Read the model definition and answer for the solid it produces. Units are mm, in the model's axes. A direction names the side the tool comes from. Coordinates: 2 decimals unless noted, no trailing zeros. Loops run counter-clockwise (first coordinate to the right, second up) from the corner with the lowest first, then second, coordinate; pieces in that order, holes last. Notation, with made-up numbers: (62.5, 75) -> (110.5, 75) arc R28 ccw to (110.5, 108) -> close; hole circle Ø6 at (4, 2). An arc over 180 degrees is marked (long way). Answer in a Markdown table with one row per item.
```python
from build123d import *

# Parameters (mm, degrees)
EXTRUDE_1_DEPTH = 6.5
SKETCH_2_R      = 8.75
EXTRUDE_2_DEPTH = 3
SKETCH_3_R      = 10
EXTRUDE_3_DEPTH = 12.5
CHAMFER_1_SIZE  = 1.5


with BuildPart() as part:
    # 草图1 → 凸台-拉伸1 (new body)
    with BuildSketch(Plane(origin=(0, 0, 0), x_dir=(1, 0, 0), z_dir=(0, 1, 0))):
        Polygon((6.553289027, 11.549360859), (-6.725395388, 11.449995205), (-13.278684415, -0.099365654), (-6.553289027, -11.549360859), (6.725395388, -11.449995205), (13.278684415, 0.099365654), align=None)
    extrude(amount=EXTRUDE_1_DEPTH)

    # 草图2 → 凸台-拉伸2 (add)
    with BuildSketch(Plane(origin=(0, 6.5, 0), x_dir=(1, 0, 0), z_dir=(0, 1, 0))):
        with Locations(Location((0, 0, 0), (0, 0, 270))):
            Circle(SKETCH_2_R)
    extrude(amount=EXTRUDE_2_DEPTH)

    # 草图3 → 凸台-拉伸3 (add)
    with BuildSketch(Plane(origin=(0, 9.5, 0), x_dir=(1, 0, 0), z_dir=(0, 1, 0))):
        with Locations(Location((0, 0, 0), (0, 0, 270))):
            Circle(SKETCH_3_R)
    extrude(amount=EXTRUDE_3_DEPTH)

    # 倒角1
    chamfer_1_edges = [part.edges().sort_by_distance(p)[0] for p in [
        (0, 22, -10),
    ]]
    chamfer(chamfer_1_edges, length=CHAMFER_1_SIZE)

    # 草图5 → 切除-旋转3 (revolve, cut)
    with BuildSketch(Plane(origin=(0, 0, 0), x_dir=(0.49350563267132574, 0, -0.8697426001534446), z_dir=(0.8697426001534445, 0, 0.4935056326713257)), mode=Mode.PRIVATE) as cut_revolve_3_sk:
        Polygon((13.279056191, 1), (11.279056191, 0), (13.279056191, 0), align=None)
    revolve(cut_revolve_3_sk.sketch.rotate(Axis((0, -1000, 0), (0, 1, 0)), 180.000000003), axis=Axis((0, -1000, 0), (0, 1, 0)), mode=Mode.SUBTRACT)


solid = part.part
```
1. The mould has two halves that part along Y. Classify faces 1 (the flat face through (0, 22, 0)), 2 (the flat face through (-9.956, 3.261, -5.756)), 3 (the flat face through (-9, 9.5, 0)): pulls with the +Y half, pulls with the -Y half, needs draft (parallel to the pull), parting line crosses it, or undercut.
A:
| item | result |
|---|---|
| face 1 | pulls with the +Y half |
| face 2 | needs draft |
| face 3 | undercut |
2. A cutting plane is placed at B-B on y = 1.5. Give the vertices of the cut face in (x, z), and give its area (3 significant figures).
A:
| item | result |
|---|---|
| outline | (-13.28, 0.1) -> (-6.73, -11.45) -> (6.55, -11.55) -> (13.28, -0.1) -> (6.73, 11.45) -> (-6.55, 11.55) -> close |
| area | 458 mm2 |
3. A tool of negligible diameter and unlimited length cuts with its end or side. For faces 4 (the flat face through (9, 6.5, 0)), 5 (the flat face through (0, 0, 0)), 6 (the cylindrical face through (-9.76, 14.92, -2.17)), from which of +Z, -Z, +X, -X, +Y, -Y can it reach the whole face along a straight path? Write none if from no direction.
A:
| item | result |
|---|---|
| face 4 | none |
| face 5 | +Z, -Z, +X, -X, -Y |
| face 6 | +Y |
4. Find the intervals of material crossed by probe 1 along Y at (x, z) = (9, -6); probe 2 along Y at (x, z) = (4.5, 8.5); probe 3 along Z at (x, y) = (6.5, 1.5), in increasing order.
A:
| item | result |
|---|---|
| probe 1 | y = 0 to 6.5 |
| probe 2 | y = 0 to 6.5, 9.5 to 20.88 |
| probe 3 | z = -11.55 to 11.45 |
5. A cutting plane is placed at A-A on x = 0. Give the vertices of the cut face in (y, z).
A:
| item | result |
|---|---|
| outline | (0, -11.28) -> (0.11, -11.5) -> (6.5, -11.5) -> (6.5, -8.75) -> (9.5, -8.75) -> (9.5, -10) -> (20.5, -10) -> (22, -8.5) -> (22, 8.5) -> (20.5, 10) -> (9.5, 10) -> (9.5, 8.75) -> (6.5, 8.75) -> (6.5, 11.5) -> (0.11, 11.5) -> (0, 11.28) -> close |
6. Given pin 1 Ø3 at (x, z) = (-10, -5) entering from +Y; pin 2 Ø6 at (y, z) = (8.5, -9) entering from +X; pin 3 Ø5 at (y, z) = (7, 2.5) entering from +X, each flat-ended and moving along its own axis, determine where each tip first touches the part or whether it passes through.
A:
| item | result |
|---|---|
| pin 1 | stops at y = 20.82 |
| pin 2 | stops at x = 9.36 |
| pin 3 | stops at x = 13.19 |
7. A cutting plane is placed at C-C on y = 9. Give the vertices of the cut face in (x, z).
A:
| item | result |
|---|---|
| outline | circle Ø17.5 at (0, 0) |
